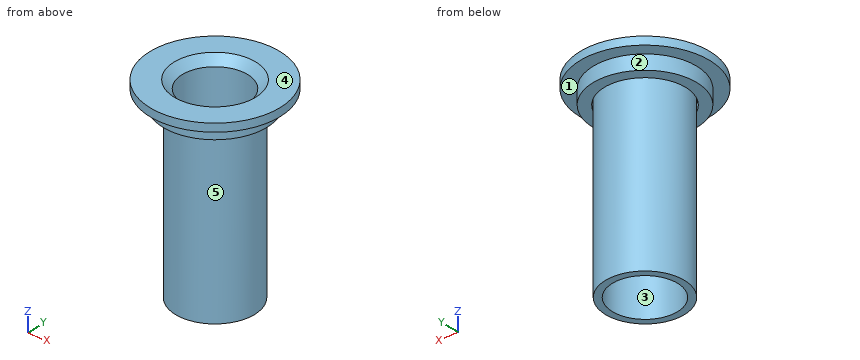
Autodesk Inventor part; units mm, degrees
ref_plane "Arbeitsebene1" through (-19.3, -19.3, 3.2) normal (0, 0, 1) x (1, 0, 0)
ref_plane "YZ Plane" through (0, 0, 0) normal (1, 0, 0) x (0, 1, 0)
ref_plane "XZ Plane" through (0, 0, 0) normal (0, 1, 0) x (-1, 0, 0)
sketch "Skizze1" plane through (0, 0, 0) normal (0, 0, 1) x (1, 0, 0)
  arc A0 (-2.8009, 5.3061) -> (2.8009, 5.3061) centre (0, 0) ccw
  circle A1 centre (0, 0) radius 5
  circle A2 centre (0, 0) radius 4.9
  circle A3 centre (0, 0) radius 4.05
  point P0 (0, 0)
  dimension "d0" = 0.1
  dimension "d1" = 8.1
extrude "Extrusion1" add sketch "Skizze1" along normal blind 6 and the other way blind 18 contours A2
sketch "Skizze2" plane through (0, 0, 6) normal (0, 0, 1) x (1, 0, 0)
  circle A0 centre (0, 0) radius 4.9
  circle A1 centre (0, 0) radius 8.5508
  circle A2 centre (0, 0) radius 7.7
  circle A3 centre (0, 0) radius 8.0508
  point P0 (0, 0)
  dimension "d4" = 0.5
extrude "Extrusion2" add sketch "Skizze2" against normal blind 1 contours A2 | A3
chamfer "Fase1" distance 1 angle 45 2 edges at (-4.9, 0, 5) (-4.05, 0, 6)
sketch "Skizze3" plane through (0, 0, 5) normal (0, 0, -1) x (-1, 0, 0)
  circle A0 centre (0, 0) radius 4.9
  circle A1 centre (0, 0) radius 5.05
  circle A2 centre (0, 0) radius 4.1058
  circle A3 centre (0, 0) radius 6.4267
  point P0 (0, 0)
ref_plane "Arbeitsebene1" through (-19.3, -19.3, 3.2) normal (0, 0, 1) x (1, 0, 0)
extrude "Extrusion3" add sketch "Skizze3" along normal up to surface (1.8 mm away)
properties part number "50_ETL_Motionpart1_v0"
CAD build for the part. Positions are in the model's coordinates, mm. Face numbers are marked on the shaded views. A direction names the side the tool comes from. Round coordinates to 2 decimals unless told otherwise and drop trailing zeros. Order: outer loops, then holes, each group sorted by start corner. A loop starts at its lowest first (then second) coordinate and runs counter-clockwise, first axis right, second up.
Q1. Which spindle directions (+Z, -Z, +X, -X, +Y, -Y) get a long thin tool onto all of the face, cutting with end or side? Do the marked faces 4 and 5. Say none if no direction does.
Q2. Drop flat-ended pins along their axis: pin 1 (2 mm diameter, centred on y = -1.5, z = -11.5, fed in from -X); pin 2 (8 mm diameter, centred on y = -5, z = -15.5, fed in from -X); pin 3 (6 mm diameter, centred on x = 1, z = -13.5, fed in from +Y). Give the stop position or say it passes through.
Q3. Slice it at B-B (x = -7). Write the cut outline in (y, z), and give its area (3 significant figures).
Q4. Two-plate mould, pull along X, no slides. Class the marked faces 1, 2 and 3: pulls with the +X half, pulls with the -X half, needs draft (parallel to the pull), parting line crosses it, or undercut.
Q5. Wall check: L1, parallel to Y at x = 0, z = -8.75; L2, parallel to Y at x = -1.5, z = 3.75. Give the ranges that are in metal, low to high.
Q6. Slice it at A-A (z = -16). Write the cut outline in (x, y), and give its area (3 significant figures).
Results below:
1. face 4: +Z, +X, -X, +Y, -Y
1. face 5: -Z
2. pin 1: stops at x = -4.87
2. pin 2: stops at x = -4.8
2. pin 3: stops at y = 4.9
3. outline: (-3.98, 5) - (3.98, 5) - (3.98, 6) - (-3.98, 6) - close
3. area: 7.95 mm2
4. face 1: needs draft
4. face 2: parting line crosses it
4. face 3: undercut
5. L1: y = -4.9 to -4.05, 4.05 to 4.9
5. L2: y = -6.25 to -4.82, -4.66 to -3.76, 3.76 to 4.66, 4.82 to 6.25
6. outline: circle Ø9.8 at (0, 0); hole circle Ø8.1 at (0, 0)
6. area: 23.9 mm2
